Geometry check sheet. Reference: the model listing, model coordinates, mm. Face numbers are marked on the shaded views. A direction names the side the tool comes from. Round coordinates to 2 decimals unless told otherwise and drop trailing zeros. Order: outer loops, then holes, each group sorted by start corner. A loop starts at its lowest first (then second) coordinate and runs counter-clockwise, first axis right, second up.
(1) Material ranges on line 1 along Y through (x, z) = (1, 34.5); line 2 along Y through (x, z) = (1.3, 36); line 3 along Y through (x, z) = (0.25, -0.5), recorded low to high.
(2) Set-up check for the marked faces 1, 2 and 3: record each of +Z, -Z, +X, -X, +Y, -Y from which the full face is reachable in a straight line by a thin tool's end or side.
(3) Sectioned sample at D-D (x = 2.75). Give the number of separate pieces and of enclosed holes in the cut face, plus the area to 3 significant figures.
(4) Go/stop test with flat-tipped pins: pin 1 (4.5 mm diameter, centred on y = 11, z = 10.5, fed in from +X); pin 2 (1 mm diameter, centred on x = 2, y = 66, fed in from +Z); pin 3 (2.5 mm diameter, centred on x = 2, y = -2, fed in from +Z); pin 4 (1.5 mm diameter, centred on x = 1.5, y = 39, fed in from -Z). Record where each tip stops, or that it passes through.
(5) Sectioned sample at C-C (z = 46.5). Record the boundary of the cut face in (x, y), plus the area to 3 significant figures.
(6) Sectioned sample at A-A (z = 34.5). Record the boundary of the cut face in (x, y).
(7) Sectioned sample at B-B (y = 11). Record the boundary of the cut face in (x, z).
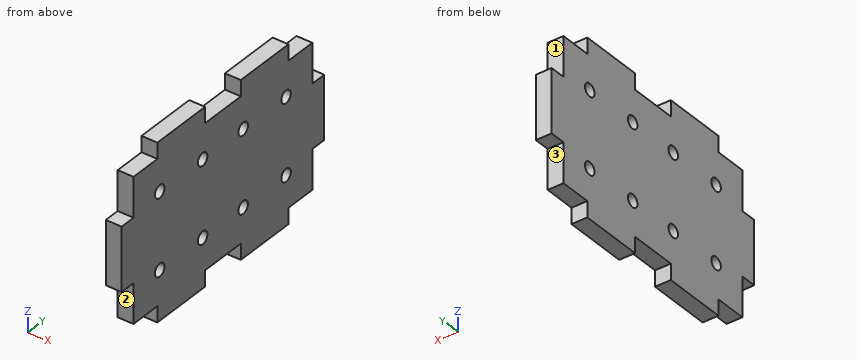
from build123d import *

# Parameters (mm, degrees)
SKETCH_1_R      = 2
EXTRUDE_1_DEPTH = 5


with BuildPart() as part:
    # 草图1 → 凸台-拉伸1 (new body)
    with BuildSketch(Plane(origin=(0, 0, 0), x_dir=(0, 0, -1), z_dir=(1, 0, 0))):
        Polygon((-32.5, 75), (-45, 75), (-45, 65), (-50, 65), (-50, 45), (-45, 45), (-45, 30), (-50, 30), (-50, 10), (-45, 10), (-45, 0), (-32.5, 0), (-32.5, -5), (-12.5, -5), (-12.5, 0), (0, 0), (0, 10), (5, 10), (5, 30), (0, 30), (0, 45), (5, 45), (5, 65), (0, 65), (0, 75), (-12.5, 75), (-12.5, 80), (-32.5, 80), align=None)
        with Locations((-34.5, 64)):
            Circle(SKETCH_1_R, mode=Mode.SUBTRACT)
        with Locations((-10.5, 64)):
            Circle(SKETCH_1_R, mode=Mode.SUBTRACT)
        with Locations((-34.5, 46)):
            Circle(SKETCH_1_R, mode=Mode.SUBTRACT)
        with Locations((-10.5, 46)):
            Circle(SKETCH_1_R, mode=Mode.SUBTRACT)
        with Locations((-34.5, 11)):
            Circle(SKETCH_1_R, mode=Mode.SUBTRACT)
        with Locations((-10.5, 11)):
            Circle(SKETCH_1_R, mode=Mode.SUBTRACT)
        with Locations((-10.5, 29)):
            Circle(SKETCH_1_R, mode=Mode.SUBTRACT)
        with Locations((-34.5, 29)):
            Circle(SKETCH_1_R, mode=Mode.SUBTRACT)
    extrude(amount=EXTRUDE_1_DEPTH)


solid = part.part
Answer below:
1. line 1: y = 0 to 9, 13 to 27, 31 to 44, 48 to 62, 66 to 75
1. line 2: y = 0 to 9.68, 12.32 to 27.68, 30.32 to 44.68, 47.32 to 62.68, 65.32 to 75
1. line 3: y = 10 to 30, 45 to 65
2. face 1: +Z, +X, -X, +Y
2. face 2: -Z, +X, -X, -Y
2. face 3: -Z, +X, -X, +Y
3. separate pieces: 1
3. enclosed holes: 8
3. area: 3,870 mm2
4. pin 1: stops at x = 5
4. pin 2: stops at z = 45
4. pin 3: stops at z = 32.5
4. pin 4: stops at z = 0
5. outline: (0, 10) - (5, 10) - (5, 30) - (0, 30) - close; (0, 45) - (5, 45) - (5, 65) - (0, 65) - close
5. area: 200 mm2
6. outline: (0, 0) - (5, 0) - (5, 9) - (0, 9) - close; (0, 13) - (5, 13) - (5, 27) - (0, 27) - close; (0, 31) - (5, 31) - (5, 44) - (0, 44) - close; (0, 48) - (5, 48) - (5, 62) - (0, 62) - close; (0, 66) - (5, 66) - (5, 75) - (0, 75) - close
7. outline: (0, -5) - (5, -5) - (5, 8.5) - (0, 8.5) - close; (0, 12.5) - (5, 12.5) - (5, 32.5) - (0, 32.5) - close; (0, 36.5) - (5, 36.5) - (5, 50) - (0, 50) - close
